Autodesk Inventor part; units mm, degrees
ref_plane "YZ Plane" through (0, 0, 0) normal (1, 0, 0) x (0, 1, 0)
ref_plane "XZ Plane" through (0, 0, 0) normal (0, 1, 0) x (-1, 0, 0)
ref_plane "XY Plane" through (0, 0, 0) normal (0, 0, 1) x (1, 0, 0)
sketch "草圖1" plane through (0, 0, 0) normal (0, 1, 0) x (-1, 0, 0)
  point P0 (0, 0)
sketch "草圖2" plane through (0, 0, 0) normal (0, 1, 0) x (-1, 0, 0)
  line L0 (0, 0) -> (300, 0)
  line L1 (300, 0) -> (300, 210)
  line L2 (300, 210) -> (0, 210)
  line L3 (0, 210) -> (0, 0)
  dimension "d0" = 210
  dimension "d1" = 300
extrude "擠出1" add sketch "草圖2" along normal blind 2
sketch "草圖3" plane through (0, 2, 0) normal (0, 1, 0) x (1, 0, 0)
  line L0 (-280, -150) -> (-20, -150)
  line L1 (-20, -150) -> (-20, 0)
  line L2 (-20, 0) -> (-280, 0)
  line L3 (-280, 0) -> (-280, -150)
  line L4 (0, 0) -> (-300, 0)
  line L5 (-300, 0) -> (-300, -210)
  dimension "d4" = 260
  dimension "d5" = 150
  dimension "d6" = 20
extrude "擠出2" cut sketch "草圖3" against normal up to surface (2 mm away)
equation "\"d0\" = W_"
equation "\"d1\" = L_"
equation "\"d2\" = h_"
equation "\"d4\" = l_"
equation "\"d5\" = w_"
equation "\"d6\" = -0.5 * l_ + 0.5 * L_"
equation "\"d7\" = h_"
equation "\"W_\" = 210"
equation "\"L_\" = 300"
equation "\"h_\" = 2"
equation "\"w_\" = 150"
equation "\"l_\" = 260"
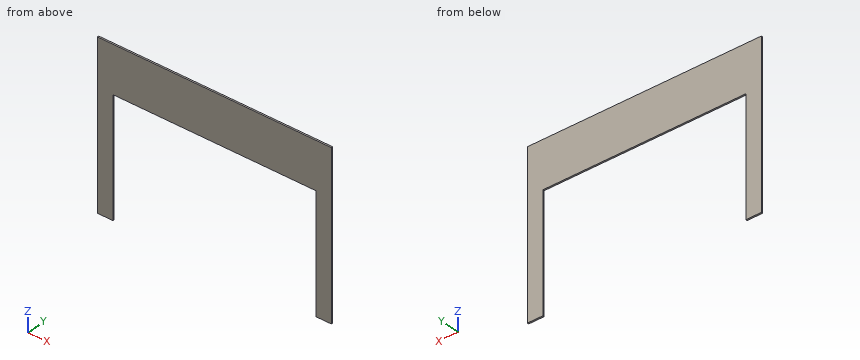
Source: CAD feature listing. Evaluate the final solid. Frame: model axes, mm. Give positions to 0.01 mm unless a question says otherwise; leave off trailing zeros. Write each loop counter-clockwise with the first axis right and the second up, starting at its lowest first coordinate (ties: lowest second). Pieces come first, ordered by that corner, then holes. Notation, with made-up numbers: M 38.5,43.25 L 64.5,43.25 A21 cw 64.5,61.25 Z; hole C 0,32.25 d5. An arc over 180 degrees is marked long. Return JSON: item names as keys, results as strings. Group by question number.
1) Cut plane B-B, the plane y = 1.45. Output: boundary loops of the cut face in (x, z), plus the area to 3 significant figures.
2) Material intervals for line 1 along X through (y, z) = (0.2, 69.5); line 2 along Z through (x, y) = (-111.5, 0.5), sorted ascending. Write a range as [from, to].
3) Pin query (flat end, axial travel): P1, Ø1, axis at x = -219.5, y = 1.5, coming from the -Z side. Return the tip coordinate at first contact, or that it passes through.
4) Cut plane C-C, the plane x = -152. Output: boundary loops of the cut face in (y, z).
5) Cut plane A-A, the plane z = 50. Output: boundary loops of the cut face in (x, y), plus the area to 3 significant figures.
Recorded:
{
 "1": {"outline": "M -300,0 L -280,0 L -280,150 L -20,150 L -20,0 L 0,0 L 0,210 L -300,210 Z", "area": "24,000 mm²"},
 "2": {"line 1": "x = [-300, -280], [-20, 0]", "line 2": "z = [150, 210]"},
 "3": {"P1": "stops at z = 150"},
 "4": {"outline": "M 0,150 L 2,150 L 2,210 L 0,210 Z"},
 "5": {"outline": "M -300,0 L -280,0 L -280,2 L -300,2 Z; M -20,0 L 0,0 L 0,2 L -20,2 Z", "area": "80.0 mm²"}
}
